Check sheet for the modelled part. Datum: model origin and axes. Units: mm. A direction names the side the tool comes from. Give positions to 0.01 mm unless a question says otherwise; leave off trailing zeros. Write each loop counter-clockwise with the first axis right and the second up, starting at its lowest first coordinate (ties: lowest second). Pieces come first, ordered by that corner, then holes. Notation, with made-up numbers: M 58,43 L 80,43 A19 cw 80,78 Z; hole C 88.5,-34 d1. An arc over 180 degrees is marked long. Write item = value, one per line. Start each with the question number.
1) Scan lines: line 1 along Y through (x, z) = (-3.7, -10); line 2 along Z through (x, y) = (-4, -39.75); line 3 along X through (y, z) = (-47.25, 3). Record each from-to range of solid material in increasing order. Write a range as [from, to].
2) Go/stop test with flat-tipped pins: pin 1 (6 mm diameter, centred on y = -42, z = -4, fed in from -X); pin 2 (1.3 mm diameter, centred on x = -7, z = 4.5, fed in from -Y); pin 3 (2 mm diameter, centred on x = -1.5, z = -2, fed in from -Y); pin 4 (4 mm diameter, centred on y = -40, z = -10, fed in from +X). Record where each tip stops, or that it passes through.
3) Mould release check, pull along Z, two halves, no side actions. Record for faces 1 (the cylindrical face through (-3.915, -37.918, -9.727)), 2 (the flat face through (-4, -32, -20)), 3 (the flat face through (-9.4, -22, 0)), 4 (the cylindrical face through (-3.915, -37.918, 10.273)): released by +Z, released by -Z, zero draft, split by the parting line, or undercut.
4) Cross-section at B-B, the plane z = 10. Record the cut outline in (x, y), plus the area to 3 significant figures.
5) Cross-section at C-C, the plane z = -1. Record the cut outline in (x, y), plus the area to 3 significant figures.
6) Cross-section at A-A, the plane y = -40. Record the cut outline in (x, z).
7) Access from +Z, -Z, +X, -X, +Y, -Y to the whole of each face (thin tool, end or side, straight path). Record for faces 5 (the flat face through (-5, -40, 0)), 6 (the flat face through (-2.8, -37, 0)), 7 (the flat face through (-4, -50, 0)), 8 (the flat face through (-5, -26, 0)).
8) Cross-section at D-D, the plane x = -6.5. Record the cut outline in (y, z).
```python
from build123d import *

# Parameters (mm, degrees)
CLIP_EXTRUDE_START           = -20
CLIP_EXTRUDE_DEPTH           = 40
ANTIOFFSETBUMP_EXTRUDE_START = -20
ANTIUPLIFTBUMP_SKETCH_W      = 0.3
ANTIUPLIFTBUMP_SKETCH_H      = 1
ANTIOFFSETBUMP_EXTRUDE_DEPTH = 40
MOUNTHOLES_CUT_DEPTH         = 55.665894029
MOUNTHOLES_CUT_DEPTH_BACK    = 55.665894029
MOUNTHOLES_SKETCH_R          = 2.1


with BuildPart() as part:
    # panelClipSection_sketch → clip_extrude (new body)
    with BuildSketch(Plane.XY.offset(CLIP_EXTRUDE_START)):
        Polygon((-9.40000037, -23.99999963), (-5.00000037, -23.99999963), (-5.00000037, -49.99999963), (-2.80000037, -49.99999963), (-2.80000037, -23.49999963), (-0.80000037, -23.49999963), (-0.80000037, -20.19999963), (-9.40000037, -20.19999963), align=None)
    extrude(amount=CLIP_EXTRUDE_DEPTH)

    # antiUpliftBump_sketch → antiOffsetBump_extrude (add)
    with BuildSketch(Plane.XY.offset(ANTIOFFSETBUMP_EXTRUDE_START)):
        with Locations((-5.15000037, -29.49999963)):
            Rectangle(ANTIUPLIFTBUMP_SKETCH_W, ANTIUPLIFTBUMP_SKETCH_H)
    extrude(amount=ANTIOFFSETBUMP_EXTRUDE_DEPTH)

    # mountHoles_sketch → mountHoles_cut (cut, two sides: drawn at the far end of the back side and taken through both)
    with BuildSketch(Plane(origin=(0, 0, 0), x_dir=(0, 0, -1), z_dir=(1, 0, 0)).offset(-MOUNTHOLES_CUT_DEPTH_BACK)):
        with Locations((10, -39.99999963)):
            Circle(MOUNTHOLES_SKETCH_R)
        with Locations((-10, -39.99999963)):
            Circle(MOUNTHOLES_SKETCH_R)
    extrude(amount=MOUNTHOLES_CUT_DEPTH + MOUNTHOLES_CUT_DEPTH_BACK, mode=Mode.SUBTRACT)


solid = part.part
```
Reply:
q1.line_1 = [-50, -42.1], [-37.9, -20.2]
q1.line_2 = [-20, -12.09], [-7.91, 7.91], [12.09, 20]
q1.line_3 = [-5, -2.8]
q2.pin_1 = -5
q2.pin_2 = -24
q2.pin_3 = -23.5
q2.pin_4 = through
q3.face_1 = undercut
q3.face_2 = released by -Z
q3.face_3 = zero draft
q3.face_4 = undercut
q4.outline = M -9.4,-24 L -5,-24 L -5,-29 L -5.3,-29 L -5.3,-30 L -5,-30 L -5,-37.9 L -2.8,-37.9 L -2.8,-23.5 L -0.8,-23.5 L -0.8,-20.2 L -9.4,-20.2 Z; M -5,-50 L -2.8,-50 L -2.8,-42.1 L -5,-42.1 Z
q4.area = 79.9 mm2
q5.outline = M -9.4,-24 L -5,-24 L -5,-29 L -5.3,-29 L -5.3,-30 L -5,-30 L -5,-50 L -2.8,-50 L -2.8,-23.5 L -0.8,-23.5 L -0.8,-20.2 L -9.4,-20.2 Z
q5.area = 89.2 mm2
q6.outline = M -5,-20 L -2.8,-20 L -2.8,-12.1 L -5,-12.1 Z; M -5,-7.9 L -2.8,-7.9 L -2.8,7.9 L -5,7.9 Z; M -5,12.1 L -2.8,12.1 L -2.8,20 L -5,20 Z
q7.face_5 = +Z, -Z, -X, -Y
q7.face_6 = +Z, -Z, +X, -Y
q7.face_7 = +Z, -Z, +X, -X, -Y
q7.face_8 = +Z, -Z, -X
q8.outline = M -24,-20 L -20.2,-20 L -20.2,20 L -24,20 Z
